Source: CAD feature listing. Evaluate the final solid. Frame: model axes, mm. Face numbers are marked on the shaded views. A direction names the side the tool comes from. Give positions to 0.01 mm unless a question says otherwise; leave off trailing zeros. Order: outer loops, then holes, each group sorted by start corner. A loop starts at its lowest first (then second) coordinate and runs counter-clockwise, first axis right, second up.
```python
from build123d import *

# Parameters (mm, degrees)
P_IDAT_VYSUNUT_M1_DEPTH  = 6
SKICA2_W                 = 6
SKICA2_H                 = 6
ODEBRAT_VYSUNUT_M1_DEPTH = 3.5
SKICA3_R                 = 1.5
ODEBRAT_VYSUNUT_M2_DEPTH = 3.5
SKICA4_W                 = 0.765185498
SKICA4_H                 = 4.384382678
SKICA4_W_2               = 0.586642215
SKICA4_W_3               = 0.510123665
P_IDAT_VYSUNUT_M2_DEPTH  = 0.2
SKICA5_W                 = 2
SKICA5_H                 = 9.5
P_IDAT_VYSUNUT_M3_DEPTH  = 2
SKICA6_R                 = 1
P_IDAT_VYSUNUT_M4_DEPTH  = 1.8
ZAOBLIT1_R               = 2.5


with BuildPart() as part:
    # Skica1 → Přidat vysunutím1 (new body)
    with BuildSketch(Plane.XY):
        Polygon((0, 0), (0, 12.5), (11, 12.5), (11, 10.5), (17, 10.5), (17, 4.5), (11, 4.5), (11, 0), align=None)
    extrude(amount=P_IDAT_VYSUNUT_M1_DEPTH)

    # Skica2 → Odebrat vysunutím1 (cut)
    with BuildSketch(Plane.XY.offset(6)):
        with Locations((14, 7.5)):
            Rectangle(SKICA2_W, SKICA2_H)
    extrude(amount=-ODEBRAT_VYSUNUT_M1_DEPTH, mode=Mode.SUBTRACT)

    # Skica3 → Odebrat vysunutím2 (cut)
    with BuildSketch(Plane.XY.offset(2.5)):
        with Locations((14, 7.5)):
            Circle(SKICA3_R)
    extrude(amount=-ODEBRAT_VYSUNUT_M2_DEPTH, mode=Mode.SUBTRACT)

    # Skica4 → Přidat vysunutím2 (add)
    with BuildSketch(Plane(origin=(0, 0, 0), x_dir=(-1, 0, 0), z_dir=(0, 0, -1))):
        with Locations((-10.040395208, -2.192191339)):
            Rectangle(SKICA4_W, SKICA4_H)
        with Locations((-5.513047674, -2.192191339)):
            Rectangle(SKICA4_W_2, SKICA4_H)
        with Locations((-0.934687773, -2.192191339)):
            Rectangle(SKICA4_W_3, SKICA4_H)
    extrude(amount=-P_IDAT_VYSUNUT_M2_DEPTH)

    # Skica5 → Přidat vysunutím3 (add)
    with BuildSketch(Plane.XY.offset(5)):
        with Locations((5.5, 17.25)):
            Rectangle(SKICA5_W, SKICA5_H)
        Polygon((7.6264998, 12.089987604), (13.732982092, 19.367409813), (15.265070979, 18.081834594), (9.158588687, 10.804412384), align=None)
        Polygon((1.841411313, 10.804412384), (-4.265070979, 18.081834594), (-2.732982092, 19.367409813), (3.3735002, 12.089987604), align=None)
    extrude(amount=-P_IDAT_VYSUNUT_M3_DEPTH)

    # Skica6 → Přidat vysunutím4 (add)
    with BuildSketch(Plane(origin=(0, 0, 0), x_dir=(-1, 0, 0), z_dir=(0, 0, -1))):
        with Locations((-5.5, 7.5)):
            Circle(SKICA6_R)
    extrude(amount=P_IDAT_VYSUNUT_M4_DEPTH)

    # Zaoblit1
    zaoblit1_edges = [part.edges().sort_by_distance(p)[0] for p in [
        (17, 10.5, 1.25),
        (17, 4.5, 1.25),
    ]]
    fillet(zaoblit1_edges, radius=ZAOBLIT1_R)


solid = part.part
```
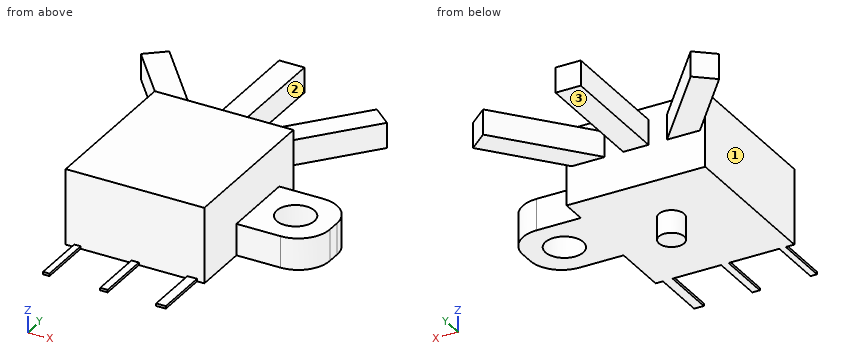
1) Section query A-A, the plane y = 7.5. Return the cut outline in (x, z).
Report:
outline: (0, 0) - (4.5, 0) - (4.5, -1.8) - (6.5, -1.8) - (6.5, 0) - (12.5, 0) - (12.5, 2.5) - (11, 2.5) - (11, 6) - (0, 6) - close; (15.5, 0) - (17, 0) - (17, 2.5) - (15.5, 2.5) - close
2) Reachability of the marked faces 1, 2 and 3 from +Z, -Z, +X, -X, +Y, -Y: full face, straight path, thin tool, end or side. Return the list, or none.
Report:
face 1: +Z, -Z, -X, -Y
face 2: +Z, -Z, +Y
face 3: -Z, +X, -X, +Y
3) Section query C-C, the plane z = 4.5. Return the cut outline in (x, y).
Report:
outline: (-4.27, 18.08) - (0.42, 12.5) - (0, 12.5) - (0, 0) - (11, 0) - (11, 12.5) - (10.58, 12.5) - (15.27, 18.08) - (13.73, 19.37) - (7.97, 12.5) - (6.5, 12.5) - (6.5, 22) - (4.5, 22) - (4.5, 12.5) - (3.03, 12.5) - (-2.73, 19.37) - close
4) Section query B-B, the plane x = 11.5. Return the cut outline in (y, z).
Report:
outline: (4.5, 0) - (10.5, 0) - (10.5, 2.5) - (4.5, 2.5) - close; (13.59, 3) - (16.71, 3) - (16.71, 5) - (13.59, 5) - close
5) Material intervals for L1, parallel to Y at x = 14, z = 1.7; L2, parallel to X at y = 13.25, z = 4.75; L3, parallel to X at y = 12.75, z = 4.25, sorted ascending.
Report:
L1: y = 4.5 to 6, 9 to 10.5
L2: x = -0.21 to 2.4, 4.5 to 6.5, 8.6 to 11.21
L3: x = 0.21 to 2.82, 4.5 to 6.5, 8.18 to 10.79
6) Pin query (flat end, axial travel): pin 1 (1 mm diameter, centred on x = 14, z = 0, fed in from +Y); pin 2 (5 mm diameter, centred on x = 14.5, y = 8, fed in from +Z); pin 3 (0.6 mm diameter, centred on x = 5, y = 16.5, fed in from +Z). Return the tip coordinate at first contact, or that it passes through.
Report:
pin 1: stops at y = 10.5
pin 2: stops at z = 2.5
pin 3: stops at z = 5
7) Section query D-D, the plane x = 5.5. Return the cut outline in (y, z), and give its area (3 significant figures).
Report:
outline: (-4.38, 0) - (6.5, 0) - (6.5, -1.8) - (8.5, -1.8) - (8.5, 0) - (12.5, 0) - (12.5, 3) - (22, 3) - (22, 5) - (12.5, 5) - (12.5, 6) - (0, 6) - (0, 0.2) - (-4.38, 0.2) - close
area: 98.5 mm2
